Design review of the part shown in the three views and the two pictorial views. Dimensions are in mm from the part's minimum x, y and z. Coordinates: 2 decimals unless noted, no trailing zeros. Loops run counter-clockwise (first coordinate to the right, second up) from the corner with the lowest first, then second, coordinate; pieces in that order, holes last. Notation, with made-up numbers: M 53,87 L 98,87 A14 ccw 98,105 Z; hole C -4,-37.5 d6. An arc over 180 degrees is marked long. Put each result on its own line as item: value. Start each with the question number.
(1) Clearance check with flat-ended pins moving along their axes: pin 1 (1.2 mm diameter, centred on y = 2, z = 23, fed in from +X); pin 2 (1.2 mm diameter, centred on y = 2.5, z = 25, fed in from -X); pin 3 (1.2 mm diameter, centred on x = 242.5, y = 2.5, fed in from +Z). State where each tip first meets the part, or that it passes through.
(2) Take a section at A-A, the plane y = 0.95. Count the separate pieces of the cut face and the enclosed holes in it, then the cut area to 3 significant figures.
(3) Take a section at B-B, the plane z = 26.5. Give the boundary of the cut face in (x, y), then the cut area to 3 significant figures.
(4) Take a section at C-C, the plane x = 79.5. Give the boundary of the cut face in (y, z).
(5) For probe 1 along X at (y, z) = (2.1, 6); probe 2 along Z at (x, y) = (4, 2.45); probe 3 along Z at (x, y) = (146, 0.95), list the stretches that pass through material, from the lowest coordinate up. Write a range as [from, to].
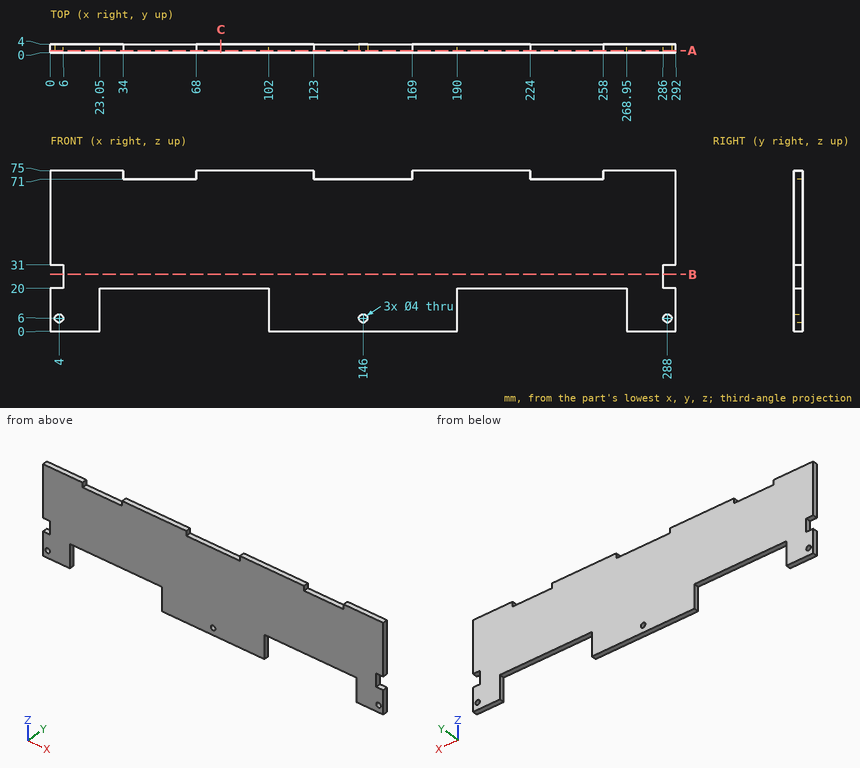
Computed values:
1. pin 1: stops at x = 286
1. pin 2: stops at x = 6
1. pin 3: stops at z = 71
2. separate pieces: 1
2. enclosed holes: 3
2. area: 18,100 mm^2
3. outline: M 6,0 L 286,0 L 286,4 L 6,4 Z
3. area: 1,120 mm^2
4. outline: M 0,20 L 4,20 L 4,75 L 0,75 Z
5. probe 1: x = [0, 2], [6, 23.05], [102, 144], [148, 190], [268.95, 286], [290, 292]
5. probe 2: z = [0, 4], [8, 20], [31, 75]
5. probe 3: z = [0, 4], [8, 71]
